Can you work these out from the model? Positions are in its coordinate system, mm. A direction names the side the tool comes from. Coordinates: 2 decimals unless noted, no trailing zeros. Write each loop counter-clockwise with the first axis right and the second up, starting at its lowest first coordinate (ties: lowest second). Pieces come first, ordered by that corner, then holes. Notation, with made-up numbers: M 1.5,-17.75 L 34.5,-17.75 A28 cw 34.5,10.25 Z; hole C 67,50 d1. An arc over 180 degrees is marked long. Use one line per item in the form item = value. Start each with the question number.
```python
from build123d import *

# Parameters (mm, degrees)
F2_W     = 10
F2_H     = 3
F3_DEPTH = 15
F4_R     = 4.99999
F5_R     = 2.5
F6_DEPTH = 18.6612540378
F7_W     = 2
F7_H     = 4.8000003753
F7_W_2   = 4.8000003753
F7_H_2   = 2
F8_DEPTH = 18


# Not quite as in the source:
# - a fillet or chamfer is up to 0.001 mm smaller than in the source, because OpenCascade refuses the exact size


with BuildPart() as f1:
    # F0 (on Top) → F1 (revolve)
    with BuildSketch(Plane.XY):
        Polygon((0, 9.2748147342), (-10, 9.2748147342), (-10, 4.304778154), (-7, 4.304778154), (-7, -14.7251852658), (-4, -14.7251852658), (-4, 4.2748147342), (0, 4.2748147342), align=None)
    revolve(axis=Axis((0, 6.7748147342, 0), (0, -1, 0)))

    # F2 (on face) → F3 (join)
    with BuildSketch(Plane(origin=(0, 9.2748147342, 0), x_dir=(-1, 0, 0), z_dir=(0, 1, 0))):
        with Locations((0, 7.1602540378)):
            Rectangle(F2_W, F2_H)
        with Locations((0, -7.1602540378)):
            Rectangle(F2_W, F2_H)
    extrude(amount=F3_DEPTH)

    # F4 (radius 5 in the source; OpenCascade refuses exactly that, so slightly less here)
    f4_edges = [f1.edges().sort_by_distance(p)[0] for p in [
        (-5, 24.274815, -7.160254),
        (5, 24.274815, -7.160254),
        (5, 24.274815, 7.160254),
        (-5, 24.274815, 7.160254),
    ]]
    fillet(f4_edges, radius=F4_R)

    # F5 (on face) → F6 (cut, through all)
    with BuildSketch(Plane(origin=(0, 0, -8.6602540378), x_dir=(1, 0, 0), z_dir=(0, 0, -1))):
        with Locations((0, -17.2748147342)):
            Circle(F5_R)
    extrude(amount=-F6_DEPTH, mode=Mode.SUBTRACT)

    # F7 (on face) → F8 (cut)
    with BuildSketch(Plane.XZ.offset(14.7251852658)):
        with Locations((0, 5.4849120788)):
            Rectangle(F7_W, F7_H)
        with Locations((-5.4849120788, 0)):
            Rectangle(F7_W_2, F7_H_2)
        with Locations((0, -5.4849120788)):
            Rectangle(F7_W, F7_H)
        with Locations((5.4849120788, 0)):
            Rectangle(F7_W_2, F7_H_2)
    extrude(amount=-F8_DEPTH, mode=Mode.SUBTRACT)


solid = f1.part
```
1) Suppose I cut it at A-A on y = 10.5. Please give me the cut outline in (x, z).
2) Will these pins go through, and if not, where does the flat tip stop? pin 1 Ø3.5 at (x, y) = (5, -6) entering from +Z; pin 2 Ø11 at (x, y) = (-1.5, 18.5) entering from -Z; pin 3 Ø1.5 at (y, z) = (16, 7.5) entering from -X; pin 4 Ø8 at (x, y) = (1.5, 2.5) entering from -Z.
3) Suppose I cut it at C-C on z = 0. Please give me the cut outline in (x, y).
4) Suppose I cut it at B-B on x = 2. Please give me the cut outline in (y, z).
5) Please list where these lines run through material, in increasing order: line 1 (Y direction, x = 0, z = 6.95); line 2 (Z direction, x = -3.75, y = 14.5); line 3 (Y direction, x = -1.25, z = -1.5).
6) If we mould it in two halves opening along X, with no side actions, what happens to faces 5 (the face through (-5, 14, 7)), 6 (the face through (-2, 15, -8.66)), 7 (the face through (0, 4.275, 0))? For each: +X half, -X half, draft (parallel to the pull), parting line (faces both ways), or undercut.
7) Which directions (+Z, -Z, +X, -X, +Y, -Y) give clear straight access to the entire face, cutting with the end or side of a thin tool? Please do faces 1 (the face through (-2, 15, 8.66)), 2 (the face through (-2, 4.305, -7)), 3 (the face through (0, 3.275, -5)), 4 (the face through (5, -6, -1)).
8) Suppose I cut it at D-D on y = -3.5. Please give me the cut outline in (x, z).
Computed values:
q1.outline = M -5,-8.66 L 5,-8.66 L 5,-5.66 L -5,-5.66 Z; M -5,5.66 L 5,5.66 L 5,8.66 L -5,8.66 Z
q2.pin_1 = 6.2
q2.pin_2 = -8.66
q2.pin_3 = -5
q2.pin_4 = -10
q3.outline = M -10,4.3 L -7,4.3 L -7,3.27 L -4,3.27 L -4,4.27 L 4,4.27 L 4,3.27 L 7,3.27 L 7,4.3 L 10,4.3 L 10,9.27 L -10,9.27 Z
q4.outline = M -14.73,-6.71 L 4.3,-6.71 L 4.3,-9.8 L 9.27,-9.8 L 9.27,-8.66 L 15.77,-8.66 L 15.77,-5.66 L 9.27,-5.66 L 9.27,5.66 L 15.77,5.66 L 15.77,8.66 L 9.27,8.66 L 9.27,9.8 L 4.3,9.8 L 4.3,6.71 L -14.73,6.71 L -14.73,3.46 L 4.27,3.46 L 4.27,-3.46 L -14.73,-3.46 Z; M 18.77,-8.66 L 23.86,-8.66 L 23.86,-5.66 L 18.77,-5.66 Z; M 18.77,5.66 L 23.86,5.66 L 23.86,8.66 L 18.77,8.66 Z
q5.line_1 = 3.27 to 14.77, 19.77 to 24.27
q5.line_2 = -8.66 to -5.66, 5.66 to 8.66
q5.line_3 = 4.27 to 9.27
q6.face_5 = -X half
q6.face_6 = draft
q6.face_7 = undercut
q7.face_1 = +Z, +X, -X, +Y
q7.face_2 = -Y
q7.face_3 = +Z, -Z, -Y
q7.face_4 = +X, -X, -Y
q8.outline = M -6.93,-1 A7 ccw -1,-6.93 L -1,-3.87 A4 cw -3.87,-1 Z; M -6.93,1 L -3.87,1 A4 cw -1,3.87 L -1,6.93 A7 ccw Z; M 1,-6.93 A7 ccw 6.93,-1 L 3.87,-1 A4 cw 1,-3.87 Z; M 1,3.87 A4 cw 3.87,1 L 6.93,1 A7 ccw 1,6.93 Z
